Could you check a few things on this model? Use its own coordinates, in mm. Round coordinates to 2 decimals unless told otherwise and drop trailing zeros. Write each loop counter-clockwise with the first axis right and the second up, starting at its lowest first coordinate (ties: lowest second). Pieces come first, ordered by that corner, then holes. Notation, with made-up numbers: M 16.25,31 L 23.25,31 A29 ccw 23.25,60 Z; hole C 47,-18 d6. An arc over 180 degrees is marked long. One line per question, with ' | ' between items. Start each with the question number.
Solid Edge part; units mm, degrees
sketch "Sketch1" plane through (0, 0, 439) normal (0, 0, 1) x (1, 0, 0)
  line L0 (-315.7, 48.875) -> (-342.9, 48.875)
  line L1 (-342.9, 48.875) -> (-342.9, 46.875)
  line L2 (-304.3, 46.875) -> (-342.9, 46.875)
  line L3 (-304.3, 57.725) -> (-304.3, 46.875)
  arc A0 (-305.8998, 61.6846) -> (-304.3, 57.725) centre (-310, 57.725) cw
  line L4 (-305.8998, 61.6846) -> (-308.6107, 64.4918)
  line L5 (-308.6107, 64.4918) -> (-311.3893, 64.4918)
  line L6 (-311.3893, 64.4918) -> (-314.1002, 61.6846)
  arc A1 (-315.7, 57.725) -> (-314.1002, 61.6846) centre (-310, 57.725) cw
  line L7 (-315.7, 48.875) -> (-315.7, 57.725)
  arc A2 (-308.0578, 59.6006) -> (-307.3, 57.725) centre (-310, 57.725) cw
  line L8 (-307.3, 57.725) -> (-307.3, 53.725)
  line L9 (-312.7, 57.725) -> (-312.7, 53.725)
  line L10 (-310, 61.6118) -> (-311.9422, 59.6006)
  line L11 (-308.0578, 59.6006) -> (-310, 61.6118)
  arc A3 (-307.3, 53.725) -> (-312.7, 53.725) centre (-310, 53.725) cw
  arc A4 (-312.7, 57.725) -> (-311.9422, 59.6006) centre (-310, 57.725) cw
extrude "ExtrudedProtrusion_1" add sketch "Sketch1" along normal blind 2
sketch "Sketch2" plane through (-323.6, 55.15, 441) normal (0, 0, 1) x (0, 1, 0)
  line L0 (-6.275, -19.3) -> (-6.275, 19.3)
  line L1 (-6.275, 19.3) -> (-8.275, 19.3)
  line L2 (-8.275, 19.3) -> (-8.275, -19.3)
  line L3 (-8.275, -19.3) -> (-6.275, -19.3)
extrude "ExtrudedProtrusion_2" add sketch "Sketch2" against normal blind 35
sketch "Sketch3" plane through (-323.6, 46.875, 419) normal (0, -1, 0) x (1, 0, 0)
  line L0 (-19.3, -13) -> (-9.3, -13)
  line L1 (-9.3, -13) -> (-9.3, -3)
  arc A0 (-9.3, -3) -> (5.7, 12) centre (5.7, -3) cw
  line L2 (5.7, 12) -> (19.3, 12)
extrude "Cutout1" cut sketch "Sketch3" against normal through all material side at (-337.9, 46.875, 405.95)
sketch "Sketch4" plane through (-323.6, 55.15, 441) normal (0, 0, 1) x (-1, 0, 0)
  line L0 (-9.5695, -6.6055) -> (3.311, 6.275)
  line L1 (-7.9, 6.275) -> (3.311, 6.275)
  line L2 (-7.9, -2.575) -> (-7.9, 6.275)
  arc A0 (-9.5695, -6.6055) -> (-7.9, -2.575) centre (-13.6, -2.575) ccw
extrude "ExtrudedProtrusion_5" add sketch "Sketch4" against normal blind 2
sketch "Sketch5" plane through (-318.3, 52.3, 429) normal (1, 0, 0) x (0, 0, -1)
  line L0 (-10, -3.425) -> (-10, -0.425)
  line L1 (-10, -0.425) -> (-7, -3.425)
  line L2 (-7, -3.425) -> (-10, -3.425)
extrude "ExtrudedProtrusion_6" add sketch "Sketch5" against normal blind 5 and the other way blind 3
properties material "ABS Plastic, medium impact"
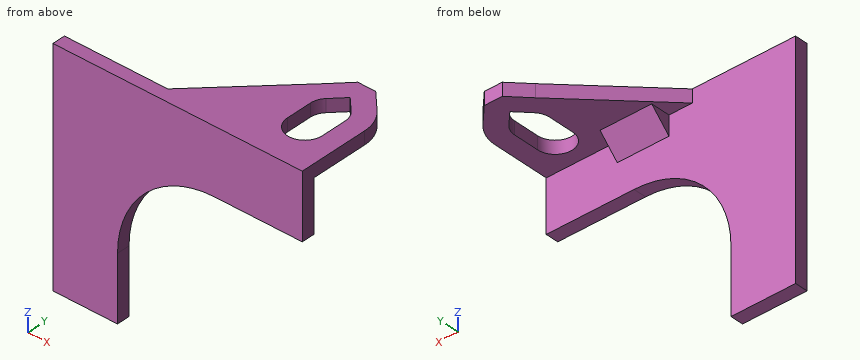
1. Suppose I cut it at C-C (z = 413). Write out the boundary of the cut face in (x, y) (3 decimals), and give its area (3 significant figures).
2. I'm going to push flat-ended pins straight in: P1, Ø1, axis at y = 48.5, z = 409.5, coming from the +X side; P2, Ø0.6, axis at y = 55.5, z = 440, coming from the -X side; P3, Ø12, axis at x = -317, z = 434, coming from the +Y side. Where does each tip first touch, or does it pass through?
3. Suppose I cut it at A-A (y = 56.25). Write out the boundary of the cut face in (x, z), and give its area (3 significant figures).
4. Suppose I cut it at B-B (y = 50). Write out the boundary of the cut face in (x, z) (3 decimals).
5. I need wall thicknesses on line 1 along Y through (x, z) = (-337, 437.5) (3 decimals); line 2 along Z through (x, y) = (-313.5, 59.25); line 3 along Z through (x, y) = (-324, 48). Which ranges of each line are inside material? Lowest first, please. Write a range as from..to.
6. Suppose I cut it at D-D (z = 423.5). Write out the boundary of the cut face in (x, y) (3 decimals).
Computed:
1) outline: M -342.9,46.875 L -332.9,46.875 L -332.9,48.875 L -342.9,48.875 Z | area: 20.0 mm²
2) P1: stops at x = -332.9 | P2: stops at x = -320.59 | P3: stops at y = 62.12
3) outline: M -319.54,439 L -312.7,439 L -312.7,441 L -319.54,441 Z; M -307.3,439 L -304.3,439 L -304.3,441 L -307.3,441 Z | area: 19.7 mm²
4) outline: M -325.786,439 L -323.3,439 L -323.3,437.125 L -315.3,437.125 L -315.3,439 L -304.3,439 L -304.3,441 L -325.786,441 Z
5) line 1: y = 46.875..48.875 | line 2: z = 439..441 | line 3: z = 429.7..441
6) outline: M -342.9,46.875 L -330.89,46.875 L -330.89,48.875 L -342.9,48.875 Z
